from build123d import *

# Parameters (mm, degrees)
SKETCH1_R      = 2.15
SKETCH1_R_2    = 8
EXTRUDE1_DEPTH = 3


with BuildPart() as part:
    # Sketch1 → Extrude1 (new body)
    with BuildSketch(Plane.XY):
        with BuildLine():
            Line((-65.365803698, -264.741816005), (-65.365803698, -284.741816005))
            Line((-65.365803698, -284.741816005), (-29.77018823, -293.224277878))
            ThreePointArc((-29.77018823, -293.224277878), (-25.365803698, -293.741816005), (-20.961419166, -293.224277878))
            Line((-20.961419166, -293.224277878), (14.634196302, -284.741816005))
            Line((14.634196302, -284.741816005), (14.634196302, -264.741816005))
            Line((14.634196302, -264.741816005), (-20.961419166, -256.259354131))
            ThreePointArc((-20.961419166, -256.259354131), (-25.365803698, -255.741816005), (-29.77018823, -256.259354131))
            Line((-29.77018823, -256.259354131), (-65.365803698, -264.741816005))
        make_face()
        with Locations((-57.365803698, -274.741816005)):
            Circle(SKETCH1_R, mode=Mode.SUBTRACT)
        with Locations((-37.365803698, -274.741816005)):
            Circle(SKETCH1_R, mode=Mode.SUBTRACT)
        with Locations((-13.365803698, -274.741816005)):
            Circle(SKETCH1_R, mode=Mode.SUBTRACT)
        with Locations((6.634196302, -274.741816005)):
            Circle(SKETCH1_R, mode=Mode.SUBTRACT)
        with Locations((-25.365803698, -274.741816005)):
            Circle(SKETCH1_R_2, mode=Mode.SUBTRACT)
        with Locations((-25.365803698, -262.741816005)):
            Circle(SKETCH1_R, mode=Mode.SUBTRACT)
        with Locations((-25.365803698, -286.741816005)):
            Circle(SKETCH1_R, mode=Mode.SUBTRACT)
    extrude(amount=EXTRUDE1_DEPTH)


solid = part.part
Geometry: final body of the model. Coordinates: model frame, mm. Give positions to 0.01 mm unless a question says otherwise; leave off trailing zeros. Loops run counter-clockwise (first coordinate to the right, second up) from the corner with the lowest first, then second, coordinate; pieces in that order, holes last. Notation, with made-up numbers: M 65,-19.75 L 110,-19.75 A9 ccw 110,-4.75 Z; hole C 10.25,-13 d5. An arc over 180 degrees is marked long. Put each result on its own line as item: value. Start each with the question number.
1) Cut plane D-D (z = 1.4). Output: boundary loops of the cut face in (x, y), then the cut area to 3 significant figures.
2) Cut plane A-A (x = -12). Output: boundary loops of the cut face in (y, z), then the cut area to 3 significant figures.
3) Contact query for a flat-ended pin moving along its axis: pin 1 (13 mm diameter, centred on x = -25.37, y = -274.74, fed in from +Z). Output: stop coordinate, or through.
4) Cut plane B-B (y = -268). Output: boundary loops of the cut face in (x, z).
5) Ray query, line 1 along X through (y, z) = (-275, 1.25); line 2 along X through (y, z) = (-279, 2.4); line 3 along X through (y, z) = (-270, 0.85). Return the intervals inside material, ascending.
6) Pull-direction query (X, two-part tool) for faces 1 (the flat face through (14.634, -275, 1)), 2 (the flat face through (-26, -266, 3)), 3 (the cylindrical face through (6.35, -272.61, 1.48)), 4 (the cylindrical face through (-25.65, -260.61, 1.48)); classes: pulls with the +X half, pulls with the -X half, needs draft (parallel to the pull), parting line crosses it, or undercut.
7) Cut plane C-C (x = -26). Output: boundary loops of the cut face in (y, z).
Verdict:
1. outline: M -65.37,-284.74 L -29.77,-293.22 A19 ccw -20.96,-293.22 L 14.63,-284.74 L 14.63,-264.74 L -20.96,-256.26 A19 ccw -29.77,-256.26 L -65.37,-264.74 Z; hole C -57.37,-274.74 d4.3; hole C -37.37,-274.74 d4.3; hole C -25.37,-274.74 d16; hole C -25.37,-286.74 d4.3; hole C -25.37,-262.74 d4.3; hole C -13.37,-274.74 d4.3; hole C 6.63,-274.74 d4.3
1. area: 2,070 mm2
2. outline: M -291.09,0 L -276.4,0 L -276.4,3 L -291.09,3 Z; M -273.08,0 L -258.39,0 L -258.39,3 L -273.08,3 Z
2. area: 88.1 mm2
3. pin 1: through
4. outline: M -65.37,0 L -29.67,0 L -29.67,3 L -65.37,3 Z; M -21.06,0 L 14.63,0 L 14.63,3 L -21.06,3 Z
5. line 1: -65.37 to -59.5, -55.23 to -39.5, -35.23 to -33.36, -17.37 to -15.5, -11.23 to 4.5, 8.77 to 14.63
5. line 2: -65.37 to -32.14, -18.59 to 14.63
5. line 3: -65.37 to -31.81, -18.92 to 14.63
6. face 1: pulls with the +X half
6. face 2: needs draft
6. face 3: undercut
6. face 4: undercut
7. outline: M -293.73,0 L -288.8,0 L -288.8,3 L -293.73,3 Z; M -284.69,0 L -282.72,0 L -282.72,3 L -284.69,3 Z; M -266.77,0 L -264.8,0 L -264.8,3 L -266.77,3 Z; M -260.69,0 L -255.75,0 L -255.75,3 L -260.69,3 Z
